Autodesk Inventor part; units mm, degrees
ref_plane "우측면도" through (0, 0, 0) normal (1, 0, 0) x (0, 1, 0)
ref_plane "평면도" through (0, 0, 0) normal (0, 1, 0) x (-1, 0, 0)
ref_plane "정면도" through (0, 0, 0) normal (0, 0, 1) x (1, 0, 0)
sketch "스케치1" plane through (0, 0, 0) normal (0, 1, 0) x (-1, 0, 0)
  line L0 (-20.5, 15) -> (20.5, 15)
  line L1 (20.5, 15) -> (20.5, -15)
  line L2 (20.5, -15) -> (-20.5, -15)
  line L3 (-20.5, -15) -> (-20.5, 15)
  line L4 (-20.5, 15) -> (20.5, -15) construction
  line L5 (20.5, 15) -> (-20.5, -15) construction
  line L6 (9, -15) -> (-9, -15)
  line L7 (9, 15) -> (-9, 15)
  line L8 (20.5, -3) -> (20.5, 15)
  line L9 (-20.5, -3) -> (-20.5, 15)
  line L10 (20.5, 6) -> (26.5, 6)
  line L11 (26.5, 6) -> (26.5, -6)
  line L12 (26.5, -6) -> (20.5, -6)
  line L13 (20.5, -6) -> (20.5, 6)
  line L14 (-20.5, 6) -> (-26.5, 6)
  line L15 (-26.5, 6) -> (-26.5, -6)
  line L16 (-26.5, -6) -> (-20.5, -6)
  line L17 (-20.5, -6) -> (-20.5, 6)
  point P0 (0, 0)
  dimension "d0" = 41
  dimension "d1" = 30
  dimension "d16" = 6
  dimension "d17" = 12
  dimension "d18" = 6
  dimension "d19" = 12
extrude "돌출3" add sketch "스케치1" along normal blind 6
sketch "스케치3" plane through (26.5, 0, 6) normal (1, 0, 0) x (0, 0, -1)
  circle A0 centre (18, 3) radius 1.35
  circle A1 centre (-6, 3) radius 1.35
  point P0 (6, 0)
  dimension "d22" = 2.7
  dimension "d23" = 2.7
extrude "돌출4" cut sketch "스케치3" against normal blind 100
sketch "스케치4" plane through (0, 6, 0) normal (0, 1, 0) x (1, 0, 0)
  line L0 (20.5, -10.65) -> (-20.5, -10.65)
  line L1 (20.5, -13.35) -> (-20.5, -13.35)
  line L2 (20.5, 10.65) -> (-20.5, 10.65)
  line L3 (20.5, 13.35) -> (-20.5, 13.35)
  line L4 (16, -13.35) -> (42.7, -13.35) construction
  line L5 (16, -13.35) -> (16, -10.65)
  line L6 (16, 10.65) -> (16, 13.35)
  line L7 (17.1, -14.6) -> (14.9, -14.6)
  line L8 (14.9, -14.6) -> (14.9, -9.4)
  line L9 (14.9, -9.4) -> (17.1, -9.4)
  line L10 (17.1, -9.4) -> (17.1, -14.6)
  line L11 (17.1, -14.6) -> (14.9, -9.4) construction
  line L12 (14.9, -14.6) -> (17.1, -9.4) construction
  line L13 (-17.1, -14.6) -> (-14.9, -14.6)
  line L14 (-14.9, -14.6) -> (-14.9, -9.4)
  line L15 (-14.9, -9.4) -> (-17.1, -9.4)
  line L16 (-17.1, -9.4) -> (-17.1, -14.6)
  line L17 (-17.1, -14.6) -> (-14.9, -9.4) construction
  line L18 (-14.9, -14.6) -> (-17.1, -9.4) construction
  line L19 (-14.9, 14.6) -> (-17.1, 14.6)
  line L20 (-17.1, 14.6) -> (-17.1, 9.4)
  line L21 (-17.1, 9.4) -> (-14.9, 9.4)
  line L22 (-14.9, 9.4) -> (-14.9, 14.6)
  line L23 (-14.9, 14.6) -> (-17.1, 9.4) construction
  line L24 (-17.1, 14.6) -> (-14.9, 9.4) construction
  line L25 (17.1, 9.4) -> (14.9, 9.4)
  line L26 (14.9, 9.4) -> (14.9, 14.6)
  line L27 (14.9, 14.6) -> (17.1, 14.6)
  line L28 (17.1, 14.6) -> (17.1, 9.4)
  line L29 (17.1, 9.4) -> (14.9, 14.6) construction
  line L30 (14.9, 9.4) -> (17.1, 14.6) construction
  point P0 (0, 0)
  point P1 (16, -12)
  point P2 (-16, -12)
  point P3 (-16, 12)
  point P4 (16, 12)
  dimension "d39" = 5
  dimension "d27" = 2.2
  dimension "d28" = 5.2
  dimension "d29" = 2.2
  dimension "d30" = 5.2
  dimension "d31" = 2.2
  dimension "d32" = 5.2
  dimension "d33" = 2.2
  dimension "d34" = 5.2
extrude "돌출5" cut sketch "스케치4" against normal blind 100 contours L10 L1 L5 L0 | L0 L8 L9 L10 | L5 L1 L8 L0 | L10 L7 L8 L1 | L14 L1 L16 L0 | L0 L16 L15 L14 | L14 L13 L16 L1 | L28 L25 L26 L2 | L2 L6 L3 L28 | L2 L26 L3 L6 | L3 L26 L27 L28 | L22 L21 L20 L2 | L2 L20 L3 L22 | L3 L20 L19 L22
sketch "스케치5" plane through (20.5, 0, -15) normal (0, 0, -1) x (-1, 0, 0)
  line L0 (0, 0) -> (41, 0)
  line L1 (41, 0) -> (41, 6)
  line L2 (41, 6) -> (0, 6)
  line L3 (0, 6) -> (0, 0)
  point P0 (20.5, 0)
  dimension "d37" = 41
  dimension "d38" = 6
extrude "돌출6" add sketch "스케치5" along normal blind 5
sketch "스케치6" plane through (-20.5, 0, 15) normal (0, 0, 1) x (1, 0, 0)
  line L0 (0, 0) -> (41, 0)
  line L1 (41, 0) -> (41, 6)
  line L2 (41, 6) -> (0, 6)
  line L3 (0, 6) -> (0, 0)
  point P0 (20.5, 0)
  dimension "d41" = 41
  dimension "d42" = 6
extrude "돌출7" add sketch "스케치6" along normal blind 5
sketch "스케치7" plane through (0, 6, 0) normal (0, 1, 0) x (1, 0, 0)
  line L0 (17.1, 14.6) -> (17.1, 9.4)
  line L1 (17.1, 9.4) -> (14.9, 9.4)
  line L2 (14.9, 9.4) -> (14.9, 14.6)
  line L3 (14.9, 14.6) -> (17.1, 14.6)
  line L4 (-14.9, -9.4) -> (-14.9, -14.6)
  line L5 (-14.9, -14.6) -> (-17.1, -14.6)
  line L6 (-17.1, -14.6) -> (-17.1, -9.4)
  line L7 (-17.1, -9.4) -> (-14.9, -9.4)
  line L8 (-17.1, 14.6) -> (-14.9, 14.6)
  line L9 (-14.9, 14.6) -> (-14.9, 9.4)
  line L10 (-14.9, 9.4) -> (-17.1, 9.4)
  line L11 (-17.1, 9.4) -> (-17.1, 14.6)
  line L12 (17.1, -9.4) -> (17.1, -14.6)
  line L13 (17.1, -14.6) -> (14.9, -14.6)
  line L14 (14.9, -14.6) -> (14.9, -9.4)
  line L15 (14.9, -9.4) -> (17.1, -9.4)
  line L16 (-20.5, 6) -> (-20.5, 20)
  line L17 (-20.5, 6) -> (-26.5, 6)
  line L18 (-26.5, 6) -> (-26.5, -6)
  line L19 (-26.5, -6) -> (-20.5, -6)
  line L20 (-20.5, -6) -> (-20.5, -20)
  line L21 (20.5, -20) -> (-20.5, -20)
  line L22 (20.5, -6) -> (20.5, -20)
  line L23 (20.5, -6) -> (26.5, -6)
  line L24 (26.5, -6) -> (26.5, 6)
  line L25 (26.5, 6) -> (20.5, 6)
  line L26 (20.5, 6) -> (20.5, 20)
  line L27 (-20.5, 20) -> (20.5, 20)
  circle A0 centre (-20.5, 6) radius 1
  circle A1 centre (-20.5, -6) radius 1
  circle A2 centre (20.5, 6) radius 1
  circle A3 centre (20.5, -6) radius 1
  point P0 (0, 0)
  point P1 (-21.5, -6)
  point P2 (-20.5, -7)
  point P3 (20.5, -7)
  point P4 (21.5, -6)
  point P5 (21.5, 6)
  point P6 (20.5, 7)
  point P7 (-20.5, 7)
  point P8 (-21.5, 6)
  dimension "d45" = 2
  dimension "d46" = 2
  dimension "d47" = 2
  dimension "d48" = 2
extrude "돌출9" cut sketch "스케치7" against normal blind 10 contours L17 A0 L16 | L16 A0 L17 | A2 L25 L26 | L26 L25 A2 | A1 L20 L19 | L19 L20 A1 | A3 L22 L23 | L23 L22 A3
properties part number "hand connection" material "PMMA 플라스틱"
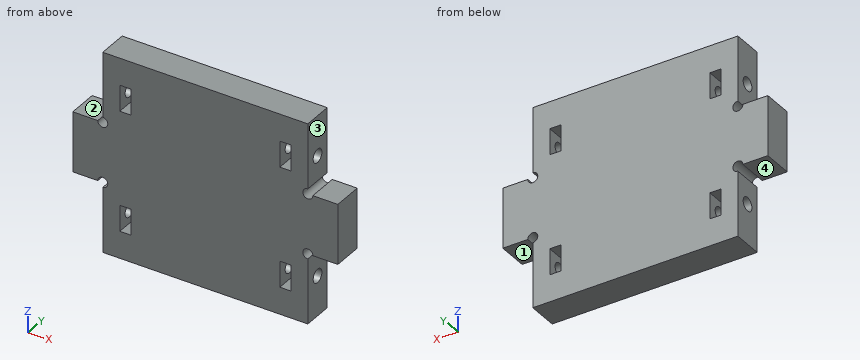
Here's how the part is built. I have some questions about the finished solid (model axes, mm). Face numbers are marked on the shaded views. A direction names the side the tool comes from. Coordinates: 2 decimals unless noted, no trailing zeros. Order: outer loops, then holes, each group sorted by start corner. A loop starts at its lowest first (then second) coordinate and runs counter-clockwise, first axis right, second up. Notation, with made-up numbers: M -13,-7.75 L -8,-7.75 A11 cw -8,10.25 Z; hole C 86,-31.5 d4. An arc over 180 degrees is marked long. Answer as a JSON object with one key per item and string values. Group by question number.
(1) Which directions (+Z, -Z, +X, -X, +Y, -Y) give clear straight access to the entire face, cutting with the end or side of a thin tool? Please do the marked faces 1, 2, 3 and 4.
(2) For pin 1 (2.5 mm diameter, centred on y = 4.5, z = -13, fed in from -X); pin 2 (2.5 mm diameter, centred on y = 2, z = -13, fed in from +X); pin 3 (2.5 mm diameter, centred on x = 24.5, y = 2, fed in from -Z); pin 4 (1.6 mm diameter, centred on y = 3, z = 12, fed in from -X), each with a flat end and sliding along its axis, tell me the tip position at first contact or that it passes through.
(3) Suppose I cut it at B-B, the plane y = 0.9. State how many separate pieces and enclosed holes the cut face has, then the cut area to 3 significant figures.
(4) Suppose I cut it at C-C, the plane x = 0. Please give me the cut outline in (y, z).
(5) Suppose I cut it at A-A, the plane z = 12. Please give me the cut outline in (x, y), then the cut area to 3 significant figures.
(6) Suppose I cut it at D-D, the plane z = 18. Please give me the cut outline in (x, y), then the cut area to 3 significant figures.
(7) I need wall thicknesses on probe 1 along Z at (x, y) = (2.5, 2.95); probe 2 along Z at (x, y) = (-17, 0.95); probe 3 along X at (y, z) = (5.35, -12). Which ranges of each line are inside material? Lowest first, please.
Values found:
{
 "1": {"face 1": "-Z, +X, +Y, -Y", "face 2": "+Z, -X, +Y, -Y", "face 3": "+Z, +X, +Y, -Y", "face 4": "-Z, -X, +Y, -Y"},
 "2": {"pin 1": "stops at x = -20.5", "pin 2": "stops at x = 20.5", "pin 3": "stops at z = -6", "pin 4": "passes through"},
 "3": {"separate pieces": "1", "enclosed holes": "4", "area": "1,730 mm^2"},
 "4": {"outline": "M 0,-20 L 6,-20 L 6,20 L 0,20 Z; hole C 3,-12 d2.7; hole C 3,12 d2.7"},
 "5": {"outline": "M -20.5,0 L -17.1,0 L -17.1,1.65 L -20.5,1.65 Z; M -20.5,4.35 L -17.1,4.35 L -17.1,6 L -20.5,6 Z; M -14.9,0 L 14.9,0 L 14.9,1.65 L -14.9,1.65 Z; M -14.9,4.35 L 14.9,4.35 L 14.9,6 L -14.9,6 Z; M 17.1,0 L 20.5,0 L 20.5,1.65 L 17.1,1.65 Z; M 17.1,4.35 L 20.5,4.35 L 20.5,6 L 17.1,6 Z", "area": "121 mm^2"},
 "6": {"outline": "M -20.5,0 L 20.5,0 L 20.5,6 L -20.5,6 Z", "area": "246 mm^2"},
 "7": {"probe 1": "z = -20 to -13.35, -10.65 to 10.65, 13.35 to 20", "probe 2": "z = -20 to -14.6, -9.4 to 9.4, 14.6 to 20", "probe 3": "x = -20.5 to -17.1, -14.9 to 14.9, 17.1 to 20.5"}
}
